Can you work these out from the model? Positions are in its coordinate system, mm. A direction names the side the tool comes from. Give positions to 0.01 mm unless a question says otherwise; leave off trailing zeros. Write each loop counter-clockwise with the first axis right and the second up, starting at its lowest first coordinate (ties: lowest second). Pieces come first, ordered by that corner, then holes. Notation, with made-up numbers: (69, 28) -> (102, 28) arc R26 cw to (102, 61) -> close; hole circle Ø5 at (24, 14.25). An arc over 180 degrees is marked (long way). Answer as CSV lines item,"result". Start each with the question number.
1. If we section it at C-C on z = 40.5: Write out the boundary of the cut face in (x, y) (3 decimals).
2. If we mould it in two halves opening along Y, with no side actions, what happens to faces 4 (the face through (4.74, 5.647, -4.375)), 5 (the face through (1.565, -11.012, 49.592))? For each: pulls with the +Y half, pulls with the -Y half, needs draft (parallel to the pull), parting line crosses it, or undercut.
3. On a 3-axis mill with a long thin cutter (end or side, diameter ignored), from which of +Z, -Z, +X, -X, +Y, -Y can I reach the whole of each face in a straight line? I mean faces 1 (the face through (7.921, -1.354, 9.253)), 2 (the face through (7.921, -1.354, -9.289)), 3 (the face through (4.74, -4.707, -2.769)). Say none if no direction works.
4. I need wall thicknesses on line 1 (X direction, y = 5, z = -37) (3 decimals); line 2 (Z direction, x = 3.5, y = 5.5); line 3 (Y direction, x = 12.75, z = -18). Which ranges of each line are inside material? Lowest first, please. Write a range as [from, to].
5. If we section it at B-B on y = -34: Write out the boundary of the cut face in (x, z) (3 decimals).
6. I'm going to push flat-ended pins straight in: P1, Ø2, axis at y = -20.5, z = -29, coming from the +X side (3 decimals); P2, Ø5.5, axis at y = 3, z = 0.5, coming from the +X side; P3, Ø2.5, axis at x = 4, y = 2, coming from the +Z side. Where does each tip first touch, or does it pass through?
Autodesk Inventor part; units mm, degrees
ref_plane "YZ Plane" through (0, 0, 0) normal (1, 0, 0) x (0, 1, 0)
ref_plane "XZ Plane" through (0, 0, 0) normal (0, 1, 0) x (-1, 0, 0)
ref_plane "XY Plane" through (0, 0, 0) normal (0, 0, 1) x (1, 0, 0)
sketch "Sketch1" plane through (0, 0, 0) normal (1, 0, 0) x (0, 1, 0)
  circle A0 centre (0, 0) radius 50.8
  dimension "d0" = 101.6
extrude "Extrusion1" add sketch "Sketch1" along normal blind 3.175
sketch "Sketch2" plane through (3.175, 0, 0) normal (1, 0, 0) x (0, 0, -1)
  circle A0 centre (0, 19.4049) radius 2.54
  point P0 (0, 0)
  dimension "d3" = 5.08
extrude "Extrusion2" add sketch "Sketch2" along normal blind 12.7 draft -10
pattern_circular "Circular Pattern1" count 10 over 360 about axis through (0, 0, 0) along (1, 0, 0) of "Extrusion2"
sketch "Sketch3" plane through (3.175, 0, 0) normal (1, 0, 0) x (0, 0, -1)
  line L0 (6.7407, 0) -> (8.0059, 2.1913)
  line L1 (8.0059, 2.1913) -> (10.5361, 2.1913)
  line L2 (10.5361, 2.1913) -> (11.8012, 0)
  line L3 (11.8012, 0) -> (10.5361, -2.1913)
  line L4 (10.5361, -2.1913) -> (8.0059, -2.1913)
  line L5 (8.0059, -2.1913) -> (6.7407, 0)
  point P0 (0, 0)
  point P1 (9.271, 0)
extrude "Extrusion3" add sketch "Sketch3" along normal blind 12.7 draft -10
pattern_circular "Circular Pattern2" count 6 over 360 about axis through (0, 0, 0) along (1, 0, 0) of "Extrusion3"
sketch "Sketch4" plane through (3.175, 0, 0) normal (1, 0, 0) x (0, 0, -1)
  line L0 (-5.461, 3.1529) -> (0, 6.3058)
  line L1 (0, 6.3058) -> (5.461, 3.1529)
  line L2 (5.461, 3.1529) -> (5.461, -3.1529)
  line L3 (5.461, -3.1529) -> (0, -6.3058)
  line L4 (0, -6.3058) -> (-5.461, -3.1529)
  line L5 (-5.461, -3.1529) -> (-5.461, 3.1529)
  line L6 (-7.0782, -4.0866) -> (0, -8.1732)
  line L7 (0, -8.1732) -> (7.0782, -4.0866)
  line L8 (7.0782, -4.0866) -> (7.0782, 4.0866)
  line L9 (7.0782, 4.0866) -> (0, 8.1732)
  line L10 (0, 8.1732) -> (-7.0782, 4.0866)
  line L11 (-7.0782, 4.0866) -> (-7.0782, -4.0866)
  point P0 (0, 0)
  point P1 (0, 0)
  dimension "d14" = 10.922
extrude "Extrusion4" add sketch "Sketch4" along normal blind 3.175
sketch "Sketch5" plane through (3.175, 0, 0) normal (1, 0, 0) x (0, 0, -1)
  circle A0 centre (0, 0) radius 3.175
  dimension "d17" = 6.35
extrude "Extrusion5" cut sketch "Sketch5" against normal through all
properties part number "foam gripper"
Computed values:
1,outline,"(0, -30.666) -> (3.175, -30.666) -> (3.175, 30.666) -> (0, 30.666) -> close"
2,face 4,"undercut"
2,face 5,"parting line crosses it"
3,face 1,"+Z, +X"
3,face 2,"-Z, +X"
3,face 3,"+X"
4,line 1,"x = [0, 3.175]"
4,line 2,"z = [-20.89, -16.02], [-4.63, -1.4], [1.4, 4.63], [16.02, 20.89]"
4,line 3,"y = [-6.72, -5.28], [5.28, 6.72]"
5,outline,"(0, -37.744) -> (3.175, -37.744) -> (3.175, 37.744) -> (0, 37.744) -> close"
6,P1,"stops at x = 3.175"
6,P2,"stops at x = 6.35"
6,P3,"stops at z = 50.79"
